Could you check a few things on this model? Use its own coordinates, in mm. Give positions to 0.01 mm unless a question says otherwise; leave off trailing zeros. Loops run counter-clockwise (first coordinate to the right, second up) from the corner with the lowest first, then second, coordinate; pieces in that order, holes last. Notation, with made-up numbers: M 59,-18 L 78,-18 A21 cw 78,19 Z; hole C -15,44.5 d7. An arc over 180 degrees is marked long. Answer in a Markdown table with one row per item. Add a question column.
1. Thinking about a two-plate mould opening in X: for faces 1 (the flat face through (-15, 48, -32)), 2 (the flat face through (0, 25, -58)), 3 (the cylindrical face through (-42.594, 23.664, -55.55)), 4 (the flat face through (-7, 41, -8)), which applies, released by +X, released by -X, zero draft, split by the parting line, or undercut?
2. If we section it at B-B on y = 10: Count the separate pieces of the cut face and the enclosed holes in it, then the cut area to 3 significant figures.
3. If we section it at A-A on y = 29.5: List the corners of the cut face in (x, z) for me, then the cut area to 3 significant figures.
4. If we section it at C-C on x = -40.5: List the corners of the cut face in (y, z) for me.
5. If we section it at D-D on z = -29.5: List the corners of the cut face in (x, y) for me.
6. I need wall thicknesses on line 1 along X through (y, z) = (18, 0); line 2 along X through (y, z) = (40.2, 0); line 3 along X through (y, z) = (45.25, 0). Which ranges of each line are inside material? Lowest first, please. Write a range as from..to.
7. I'm going to push flat-ended pins straight in: pin 1 Ø1.5 at (y, z) = (37, 27.5) entering from +X; pin 2 Ø5.5 at (y, z) = (13.5, 1) entering from -X; pin 3 Ø3.5 at (x, y) = (27.5, 37) entering from +Z. Where does each tip first touch, or does it pass through?
```python
from build123d import *

# Parameters (mm, degrees)
SKETCH1_R           = 70
BOSS_EXTRUDE1_DEPTH = 48
SKETCH2_R           = 35
CUT_EXTRUDE1_DEPTH  = 7
SKETCH3_R           = 10.25
CUT_EXTRUDE2_DEPTH  = 108.14942837
SKETCH4_R           = 65
CUT_EXTRUDE4_DEPTH  = 38
BOSS_EXTRUDE2_DEPTH = 38
CUT_EXTRUDE5_DEPTH  = 25
CIRPATTERN1_COUNT   = 4
BOSS_EXTRUDE3_DEPTH = 3


with BuildPart() as part:
    # Sketch1 → Boss-Extrude1 (new body)
    with BuildSketch(Plane(origin=(0, 0, 0), x_dir=(1, 0, 0), z_dir=(0, 1, 0))):
        with Locations(Location((0, 0, 0), (0, 0, 270))):
            Circle(SKETCH1_R)
    extrude(amount=BOSS_EXTRUDE1_DEPTH)

    # Sketch2 → Cut-Extrude1 (cut)
    with BuildSketch(Plane(origin=(0, 48, 0), x_dir=(1, 0, 0), z_dir=(0, 1, 0))):
        with Locations(Location((0, 0, 0), (0, 0, 270))):
            Circle(SKETCH2_R)
    extrude(amount=-CUT_EXTRUDE1_DEPTH, mode=Mode.SUBTRACT)

    # Sketch3 → Cut-Extrude2 (cut, through all)
    with BuildSketch(Plane(origin=(0, 41, 0), x_dir=(1, 0, 0), z_dir=(0, 1, 0))):
        with Locations(Location((0, 0, 0), (0, 0, 270))):
            Circle(SKETCH3_R)
    extrude(amount=-CUT_EXTRUDE2_DEPTH, mode=Mode.SUBTRACT)

    # Sketch4 → Cut-Extrude4 (cut)
    with BuildSketch(Plane.XZ):
        with Locations(Location((0, 0, 0), (0, 0, 270))):
            Circle(SKETCH4_R)
    extrude(amount=-CUT_EXTRUDE4_DEPTH, mode=Mode.SUBTRACT)

    # Sketch7 → Boss-Extrude2 (add)
    with BuildSketch(Plane.XZ.offset(-38)):
        Polygon((-57.5, 4.907477288), (-61.75, 2.453738644), (-61.75, -2.453738644), (-57.5, -4.907477288), (-53.25, -2.453738644), (-53.25, 2.453738644), align=None)
    boss_extrude2 = extrude(amount=BOSS_EXTRUDE2_DEPTH)

    # Sketch10 → Cut-Extrude5 (cut)
    with BuildSketch(Plane.XZ):
        Polygon((-57.5, 3.175426481), (-60.25, 1.58771324), (-60.25, -1.58771324), (-57.5, -3.175426481), (-54.75, -1.58771324), (-54.75, 1.58771324), align=None)
    cut_extrude5 = extrude(amount=-CUT_EXTRUDE5_DEPTH, mode=Mode.SUBTRACT)

    # CirPattern1: Boss-Extrude2, Cut-Extrude5 ×4 about axis
    cirpattern1_axis = Axis((0, 0, 0), (0, 1, 0))
    add([boss_extrude2.rotate(cirpattern1_axis, i * 360 / CIRPATTERN1_COUNT) for i in range(1, CIRPATTERN1_COUNT)])
    add([cut_extrude5.rotate(cirpattern1_axis, i * 360 / CIRPATTERN1_COUNT) for i in range(1, CIRPATTERN1_COUNT)], mode=Mode.SUBTRACT)

    # Sketch14 → Boss-Extrude3 (add)
    with BuildSketch(Plane.XZ.offset(-38)):
        Polygon((31.041266081, 38.890872965), (29.309215274, 41.890872965), (25.845113659, 41.890872965), (24.113062851, 38.890872965), (25.845113659, 35.890872965), (29.309215274, 35.890872965), align=None)
        Polygon((25.26776339, 38.890872965), (26.422463928, 36.890872965), (28.731865005, 36.890872965), (29.886565543, 38.890872965), (28.731865005, 40.890872965), (26.422463928, 40.890872965), align=None, mode=Mode.SUBTRACT)
    boss_extrude3 = extrude(amount=BOSS_EXTRUDE3_DEPTH)

    # Mirror1: Boss-Extrude3 across plane
    add(boss_extrude3.mirror(Plane(origin=(0, 0, 0), x_dir=(0.7071067811865436, 0, 0.7071067811865515), z_dir=(-0.7071067811865515, 0, 0.7071067811865436))))


solid = part.part
```
Results:
| question | item | result |
|---|---|---|
| 1 | face 1 | zero draft |
| 1 | face 2 | undercut |
| 1 | face 3 | split by the parting line |
| 1 | face 4 | undercut |
| 2 | separate pieces | 5 |
| 2 | enclosed holes | 5 |
| 2 | area | 2,270 mm2 |
| 3 | outline | C 0,0 d140; M -61.75,-2.45 L -57.5,-4.91 L -53.25,-2.45 L -53.25,2.45 L -57.5,4.91 L -61.75,2.45 Z; M -4.91,-57.5 L -2.45,-61.75 L 2.45,-61.75 L 4.91,-57.5 L 2.45,-53.25 L -2.45,-53.25 Z; M -4.91,57.5 L -2.45,53.25 L 2.45,53.25 L 4.91,57.5 L 2.45,61.75 L -2.45,61.75 Z; M 53.25,-2.45 L 57.5,-4.91 L 61.75,-2.45 L 61.75,2.45 L 57.5,4.91 L 53.25,2.45 Z; hole C 0,0 d130 |
| 3 | area | 2,370 mm2 |
| 4 | outline | M 0,-57.09 L 48,-57.09 L 48,57.09 L 0,57.09 L 0,50.84 L 38,50.84 L 38,-50.84 L 0,-50.84 Z |
| 5 | outline | M -63.48,0 L -57.92,0 L -57.92,38 L 57.92,38 L 57.92,0 L 63.48,0 L 63.48,48 L 18.83,48 L 18.83,41 L -18.83,41 L -18.83,48 L -63.48,48 Z |
| 6 | line 1 | -70..-65, -61.75..-60.25, -54.75..-53.25, 53.25..54.75, 60.25..61.75, 65..70 |
| 6 | line 2 | -70..-10.25, 10.25..70 |
| 6 | line 3 | -70..-35, 35..70 |
| 7 | pin 1 | x = 64.69 |
| 7 | pin 2 | x = -70 |
| 7 | pin 3 | z = 65.09 |
